Geometry: final body of the model. Coordinates: model frame, mm. A direction names the side the tool comes from. Coordinates: 2 decimals unless noted, no trailing zeros. Write each loop counter-clockwise with the first axis right and the second up, starting at its lowest first coordinate (ties: lowest second). Pieces come first, ordered by that corner, then holes.
from build123d import *

# Parameters (mm, degrees)
ESQUISSE1_R             = 61
BOSS_EXTRU_1_DEPTH      = 2
BOSS_EXTRU_2_START      = 10
ESQUISSE2_R             = 61
ESQUISSE2_R_2           = 59
BOSS_EXTRU_2_DEPTH      = 10
ESQUISSE3_R             = 3
BOSS_EXTRU_3_DEPTH      = 10
ENL_V_MAT_EXTRU_6_DEPTH = 10
ESQUISSE7_W             = 4.037056784
ESQUISSE7_H             = 1
BOSS_EXTRU_4_DEPTH      = 53


with BuildPart() as part:
    # Esquisse1 → Boss.-Extru.1 (new body)
    with BuildSketch(Plane(origin=(0, 0, 0), x_dir=(1, 0, 0), z_dir=(0, 1, 0))):
        with Locations(Location((0, 0, 0), (0, 0, 270))):
            Circle(ESQUISSE1_R)
    extrude(amount=BOSS_EXTRU_1_DEPTH)

    # Esquisse2 → Boss.-Extru.2 (add)
    with BuildSketch(Plane(origin=(0, 0, 0), x_dir=(-1, 0, 0), z_dir=(0, -1, 0)).offset(BOSS_EXTRU_2_START)):
        with Locations(Location((0, 0, 0), (0, 0, 90))):
            Circle(ESQUISSE2_R)
        with Locations(Location((0, 0, 0), (0, 0, 90))):
            Circle(ESQUISSE2_R_2, mode=Mode.SUBTRACT)
    extrude(amount=-BOSS_EXTRU_2_DEPTH)

    # Esquisse3 → Boss.-Extru.3 (add)
    with BuildSketch(Plane(origin=(0, 0, 0), x_dir=(-1, 0, 0), z_dir=(0, -1, 0))):
        with Locations(Location((0, 0, 0), (0, 0, 270))):
            Circle(ESQUISSE3_R)
    extrude(amount=BOSS_EXTRU_3_DEPTH)

    # Esquisse5 → Enlèv. mat.-Extru.6 (cut)
    with BuildSketch(Plane(origin=(0, 2, 0), x_dir=(1, 0, 0), z_dir=(0, 1, 0))):
        with BuildLine():
            ThreePointArc((-55.883459525, 1), (-39.521899299, 39.521899299), (-1, 55.883459525))
            Line((-1, 55.883459525), (-1, 2.828427125))
            ThreePointArc((-1, 2.828427125), (-2.121320344, 2.121320344), (-2.828427125, 1))
            Line((-2.828427125, 1), (-55.883459525, 1))
        make_face()
    extrude(amount=-ENL_V_MAT_EXTRU_6_DEPTH, mode=Mode.SUBTRACT)

    # Esquisse7 → Boss.-Extru.4 (add)
    with BuildSketch(Plane(origin=(0, 0, 0), x_dir=(-1, 0, 0), z_dir=(0, -1, 0))):
        with Locations((0.001904175, -2)):
            Rectangle(ESQUISSE7_W, ESQUISSE7_H)
        with BuildLine():
            Line((-2.007102857, 1.502061623), (-2.007102857, 2.5))
            Line((-2.007102857, 2.5), (1.607669388, 2.5))
            ThreePointArc((1.607669388, 2.5), (1.792908074, 2.346421898), (1.992897143, 2.212616159))
            Line((1.992897143, 2.212616159), (1.992897143, 1.502061623))
            Line((1.992897143, 1.502061623), (-2.007102857, 1.502061623))
        make_face()
    extrude(amount=BOSS_EXTRU_4_DEPTH)


solid = part.part
Item 1: Set-up query: faces 3 (the flat face through (0, -31, 1.5)), 4 (the cylindrical face through (3, -5, 0)). Return all of +Z, -Z, +X, -X, +Y, -Y with unobstructed straight access to the full face (end or side cutting, diameter ignored); none if empty.
Derived:
face 3: +X, -X, -Y
face 4: -Y
Item 2: Section D-D, the plane x = 7. Output: boundary loops of the cut face in (y, z), plus the area to 3 significant figures.
Derived:
outline: (-10, -60.6) - (2, -60.6) - (2, 60.6) - (-10, 60.6) - (-10, 58.58) - (0, 58.58) - (0, -58.58) - (-10, -58.58) - close
area: 283 mm2
Item 3: Section A-A, the plane x = -7.5. Output: boundary loops of the cut face in (y, z), plus the area to 3 significant figures.
Derived:
outline: (-10, -60.54) - (2, -60.54) - (2, -55.39) - (0, -55.39) - (0, -58.52) - (-10, -58.52) - close; (-10, 58.52) - (0, 58.52) - (0, -1) - (2, -1) - (2, 60.54) - (-10, 60.54) - close
area: 174 mm2
Item 4: Pin query (flat end, axial travel): pin 1 (10 mm diameter, centred on y = -29.5, z = -5, fed in from -X); pin 2 (3 mm diameter, centred on x = 0, y = -33.5, fed in from +Z); pin 3 (0.8 mm diameter, centred on y = -15, z = 2, fed in from +X). Return the tip coordinate at first contact, or that it passes through.
Derived:
pin 1: stops at x = -1.99
pin 2: stops at z = 2.5
pin 3: stops at x = 2.02
Item 5: Section B-B, the plane y = -24.5. Output: boundary loops of the cut face in (x, z).
Derived:
outline: (-2.02, 1.5) - (2.02, 1.5) - (2.02, 2.5) - (-2.02, 2.5) - close; (-1.99, -2.21) arc R2.35 cw to (-1.61, -2.5) - (2.01, -2.5) - (2.01, -1.5) - (-1.99, -1.5) - close
Item 6: Section C-C, the plane z = -33. Output: boundary loops of the cut face in (x, y).
Derived:
outline: (-51.3, -10) - (-48.91, -10) - (-48.91, 0) - (-45.11, 0) - (-45.11, 2) - (-51.3, 2) - close; (-1, 0) - (48.91, 0) - (48.91, -10) - (51.3, -10) - (51.3, 2) - (-1, 2) - close
Item 7: Material intervals for probe 1 along X at (y, z) = (-4, 0); probe 2 along Y at (x, z) = (27.5, -11), sorted ascending.
Derived:
probe 1: x = -61 to -59, -3 to 3, 59 to 61
probe 2: y = 0 to 2
Item 8: Pull-direction query (X, two-part tool) for faces 1 (the cylindrical face through (-39.944, 1.014, -39.095)), 2 (the flat face through (1, 2, -1)); classes: released by +X, released by -X, zero draft, split by the parting line, or undercut.
Derived:
face 1: undercut
face 2: zero draft
